from build123d import *

# Parameters (mm, degrees)
F1_DEPTH = 50.8
F2_DEPTH = 50.8
F4_T     = -2.54


with BuildPart() as f1:
    # F0 (on Front) → F1 (new body)
    with BuildSketch(Plane.XZ):
        Polygon((-85.1854681969, 35.1092815399), (-72.8762447834, 9.9313110113), (-46.8590036035, 9.9313110113), align=None)
    extrude(amount=F1_DEPTH)

    # F0 (on Front) → F2 (join)
    with BuildSketch(Plane.XZ):
        Polygon((-46.8590036035, 9.9313110113), (-72.8762447834, 9.9313110113), (-72.8762447834, 2.6576747186), (48.8172881305, 2.6576747186), (48.8172881305, 9.9313110113), align=None)
    extrude(amount=F2_DEPTH)

    # F3: F1 across plane


with BuildPart() as f1_1:
    add(f1.part)
    add(f1.part.mirror(Plane.YZ))

    # F4
    f4_openings = [f1_1.faces().sort_by_distance(p)[0] for p in [
        (-66.022236, -25.4, 22.520296),
        (79.030856, -25.4, 22.520296),
        (66.022236, -25.4, 22.520296),
        (-79.030856, -25.4, 22.520296),
        (0, -25.4, 9.931311),
        (72.876245, -25.4, 6.294493),
        (-72.876245, -25.4, 6.294493),
    ]]
    offset(amount=F4_T, openings=f4_openings)


solid = f1_1.part
Input: part model. Units: mm. Frame: model coordinates. A direction names the side the tool comes from. Give positions to 0.01 mm unless a question says otherwise; leave off trailing zeros. Write each loop counter-clockwise with the first axis right and the second up, starting at its lowest first coordinate (ties: lowest second). Pieces come first, ordered by that corner, then holes.
Q1. Material intervals for probe 1 along Y at (x, z) = (66, 13); probe 2 along Z at (x, y) = (-23, -41.5); probe 3 along X at (y, z) = (-15, 4), sorted ascending.
Q2. Set-up query: faces 4 (the face through (-72.876, -19, 5)), 5 (the face through (0, -50.8, 8)), 6 (the face through (72.876, -19, 5)), 7 (the face through (-65.75, -49.51, 22.34)), 8 (the face through (0, -48.26, 8)). Return all of +Z, -Z, +X, -X, +Y, -Y with unobstructed straight access to the full face (end or side cutting, diameter ignored); none if empty.
Q3. First-contact query: P1, Ø6, axis at y = -13, z = 6.5, coming from the -X side; P2, Ø4, axis at x = -8, y = -21.5, coming from the +Z side; P3, Ø3, axis at x = 19.5, y = -1, coming from the +Z side. Flat tips, straight axial feed; report the tip coordinate or a pass-through.
Q4. Section C-C, the plane z = 33.5. Output: boundary loops of the cut face in (x, y).
Q5. Section A-A, the plane z = 16. Output: boundary loops of the cut face in (x, y), plus the area to 3 significant figures.
Q6. Section D-D, the plane y = -38.5. Output: boundary loops of the cut face in (x, z), plus the area to 3 significant figures.
Q7. Pull-direction query (X, two-part tool) for faces 1 (the face through (-79.12, -49.51, 22.7)), 2 (the face through (0, 0, 8)), 3 (the face through (65.75, -1.25, 22.34)); classes: pulls with the +X half, pulls with the -X half, needs draft (parallel to the pull), parting line crosses it, or undercut.
Q8. Section B-B, the plane x = -45. Output: boundary loops of the cut face in (y, z), plus the area to 3 significant figures.
Filled in:
1. probe 1: y = -50.8 to -48.26, -2.54 to 0
1. probe 2: z = 2.66 to 5.2
1. probe 3: x = -72.88 to 72.88
2. face 4: -Z, -X, +Y, -Y
2. face 5: +Z, -Z, +X, -X, -Y
2. face 6: -Z, +X, +Y, -Y
2. face 7: +Z, +Y, -Y
2. face 8: +Z, +X, -X
3. P1: stops at x = -72.88
3. P2: stops at z = 5.2
3. P3: stops at z = 9.93
4. outline: (-84.4, -50.8) - (-82.74, -50.8) - (-82.74, -48.26) - (-84.4, -48.26) - close; (-84.4, -2.54) - (-82.74, -2.54) - (-82.74, 0) - (-84.4, 0) - close; (82.74, -50.8) - (84.4, -50.8) - (84.4, -48.26) - (82.74, -48.26) - close; (82.74, -2.54) - (84.4, -2.54) - (84.4, 0) - (82.74, 0) - close
5. outline: (-75.84, -50.8) - (-56.1, -50.8) - (-56.1, -48.26) - (-75.84, -48.26) - close; (-75.84, -2.54) - (-56.1, -2.54) - (-56.1, 0) - (-75.84, 0) - close; (56.1, -50.8) - (75.84, -50.8) - (75.84, -48.26) - (56.1, -48.26) - close; (56.1, -2.54) - (75.84, -2.54) - (75.84, 0) - (56.1, 0) - close
5. area: 201 mm2
6. outline: (-72.88, 2.66) - (72.88, 2.66) - (72.88, 5.2) - (-72.88, 5.2) - close
6. area: 370 mm2
7. face 1: pulls with the -X half
7. face 2: needs draft
7. face 3: undercut
8. outline: (-50.8, 2.66) - (0, 2.66) - (0, 9.93) - (-2.54, 9.93) - (-2.54, 5.2) - (-48.26, 5.2) - (-48.26, 9.93) - (-50.8, 9.93) - close
8. area: 153 mm2
